Read the model definition and answer for the solid it produces. Units are mm, in the model's axes. A direction names the side the tool comes from. Round coordinates to 2 decimals unless told otherwise and drop trailing zeros. Order: outer loops, then holes, each group sorted by start corner. A loop starts at its lowest first (then second) coordinate and runs counter-clockwise, first axis right, second up.
from build123d import *

# Parameters (mm, degrees)
SKETCH1_W           = 15
SKETCH1_H           = 15
BOSS_EXTRUDE1_DEPTH = 58.5
BOSS_EXTRUDE1_TAPER = 1.5
SKETCH2_R           = 1.5
CUT_EXTRUDE1_DEPTH  = 10
SKETCH3_R           = 2.75
CUT_EXTRUDE2_DEPTH  = 2
FILLET1_R           = 1.5
FILLET2_R           = 0.5


with BuildPart() as part:
    # Sketch1 → Boss-Extrude1 (new body)
    with BuildSketch(Plane.XY):
        Rectangle(SKETCH1_W, SKETCH1_H)
    extrude(amount=BOSS_EXTRUDE1_DEPTH, taper=BOSS_EXTRUDE1_TAPER)

    # Sketch2 → Cut-Extrude1 (cut)
    with BuildSketch(Plane(origin=(0, 0, 0), x_dir=(-1, 0, 0), z_dir=(0, 0, -1))):
        Circle(SKETCH2_R)
    extrude(amount=-CUT_EXTRUDE1_DEPTH, mode=Mode.SUBTRACT)

    # Sketch3 → Cut-Extrude2 (cut)
    with BuildSketch(Plane.XY.offset(58.5)):
        Circle(SKETCH3_R)
    extrude(amount=-CUT_EXTRUDE2_DEPTH, mode=Mode.SUBTRACT)

    # Fillet1
    fillet1_edges = [part.edges().sort_by_distance(p)[0] for p in [
        (-5.968123588, 0, 58.5),
        (0, -5.968123588, 58.5),
        (5.968123588, 0, 58.5),
        (6.734061794, -6.734061794, 29.25),
        (-6.734061794, -6.734061794, 29.25),
        (-6.734061332, 6.734061332, 29.250017641),
        (6.734061794, 6.734061794, 29.25),
        (0, 5.968123588, 58.5),
    ]]
    fillet(fillet1_edges, radius=FILLET1_R)

    # Fillet2
    fillet2_edges = [part.edges().sort_by_distance(p)[0] for p in [
        (1.5, 0, 0),
    ]]
    fillet(fillet2_edges, radius=FILLET2_R)


solid = part.part
Q1. A cutting plane is placed at A-A, the plane x = 0. Give the vertices of the cut face in (y, z), plus the area to 3 significant figures.
Outcome:
outline: (-7.5, 0) - (-2, 0) arc R0.5 ccw to (-1.5, 0.5) - (-1.5, 10) - (1.5, 10) - (1.5, 0.5) arc R0.5 ccw to (2, 0) - (7.5, 0) - (6.01, 57.04) arc R1.5 ccw to (4.51, 58.5) - (2.75, 58.5) - (2.75, 56.5) - (-2.75, 56.5) - (-2.75, 58.5) - (-4.51, 58.5) arc R1.5 ccw to (-6.01, 57.04) - close
area: 746 mm2
Q2. For faces 1 (the face through (1.5, 0.07, 5.18)), 2 (the face through (0, 0, 56.5)), 3 (the face through (0.06, -5.57, 58.06)), determine the directions among +Z, -Z, +X, -X, +Y, -Y from which every point of the face is accessible in a straight line to the end or side of a thin tool.
Outcome:
face 1: -Z
face 2: +Z
face 3: +Z, +X, -X, -Y
Q3. Straight lines are drawn through the part: probe 1 along Y at (x, z) = (0, 4.5); probe 2 along Y at (x, z) = (0, 58.05); probe 3 along Z at (x, y) = (3.75, 5). For each, find the intervals that lie inside material, in ascending order.
Outcome:
probe 1: y = -7.38 to -1.5, 1.5 to 7.38
probe 2: y = -5.58 to -2.75, 2.75 to 5.58
probe 3: z = 0 to 58.42
Q4. For a pull along Y with two mould halves and no side action, classify faces 4 (the face through (-0.06, 5.57, 58.06)), 5 (the face through (-0.596, -2.685, 57.514)), 6 (the face through (-5.57, -0.06, 58.06)) as released by +Y, released by -Y, zero draft, split by the parting line, or undercut.
Outcome:
face 4: released by +Y
face 5: undercut
face 6: zero draft
Q5. A cutting plane is placed at C-C, the plane y = -3.5. Give the vertices of the cut face in (x, z), plus the area to 3 significant figures.
Outcome:
outline: (-7.5, 0) - (7.5, 0) - (6.01, 57.04) arc R1.5 ccw to (4.51, 58.5) - (-4.51, 58.5) arc R1.5 ccw to (-6.01, 57.04) - close
area: 787 mm2
Q6. Flat-ended cylindrical pins translate along their axes: pin 1 (6 mm diameter, centred on y = 3, z = 15.5, fed in from +X); pin 2 (1 mm diameter, centred on x = -1.5, z = 35.5, fed in from +Y); pin 3 (5 mm diameter, centred on y = 4.5, z = 19, fed in from +X). Find the tip coordinate at first contact, or state that the pin passes through.
Outcome:
pin 1: stops at x = 7.17
pin 2: stops at y = 6.58
pin 3: stops at x = 7.07
